Check sheet for the modelled part. Datum: model origin and axes. Units: mm. A direction names the side the tool comes from. Round coordinates to 2 decimals unless told otherwise and drop trailing zeros. Loops run counter-clockwise (first coordinate to the right, second up) from the corner with the lowest first, then second, coordinate; pieces in that order, holes last. Notation, with made-up numbers: M 4.5,35.5 L 61.5,35.5 A16 ccw 61.5,51.5 Z; hole C 45,-5 d9. An arc over 180 degrees is marked long. Write item = value, one per line. Start each with the question number.
(1) Cross-section at A-A on y = 85. Record the boundary of the cut face in (x, z).
(2) Set-up check for faces 1 (the face through (30, 70, -25)), 2 (the face through (300, 32, -199)), 3 (the face through (59, 90, -136)): record each of +Z, -Z, +X, -X, +Y, -Y from which the full face is reachable in a straight line by a thin tool's end or side.
(3) Cross-section at D-D on y = 35.5. Record the boundary of the cut face in (x, z).
(4) Go/stop test with flat-tipped pins: P1, Ø2, axis at y = 103.5, z = -255, coming from the +X side; P2, Ø1, axis at x = 73, y = 66, coming from the +Z side; P3, Ø10, axis at y = 88.5, z = -178, coming from the +X side. Record where each tip stops, or that it passes through.
(5) Scan lines: L1, parallel to Y at x = 205, z = -243; L2, parallel to Z at x = 234.5, y = 84; L3, parallel to Z at x = 75, y = 45.5. Record each from-to range of solid material in increasing order. Write a range as from..to.
(6) Cross-section at B-B on z = -175. Record the boundary of the cut face in (x, y), plus the area to 3 significant figures.
(7) Cross-section at C-C on x = 205. Record the boundary of the cut face in (y, z).
(8) Mould release check, pull along X, two halves, no side actions. Record for faces 4 (the face through (0, 46, -152)), 5 (the face through (154, 92, -225)), 6 (the face through (78.252, 45.63, -189.643)): pulls with the +X half, pulls with the -X half, needs draft (parallel to the pull), parting line crosses it, or undercut.
Autodesk Fusion 360 part; units mm, degrees
sketch "Sketch1" plane through (0, 0, 0) normal (0, 1, 0) x (1, 0, 0)
  line L0 (0, 0) -> (300, 0)
  line L1 (300, 0) -> (300, 300)
  line L2 (300, 300) -> (0, 300)
  line L3 (0, 300) -> (0, 0)
  line L4 (0, 0) -> (200, 0)
  line L5 (300, 300) -> (300, 100)
  line L6 (200, 0) -> (300, 100)
  dimension "d1" = 300
  dimension "d2" = 300
  dimension "d3" = 200
  dimension "d4" = 200
extrude "Extrude1" add sketch "Sketch1" along normal blind 50 contours L0 L1 L2 L3 L4 L5 L6
sketch "Sketch2" plane through (0, 50, 0) normal (0, 1, 0) x (-1, 0, 0)
  line L0 (-300, -300) -> (0, -300)
  line L1 (0, -300) -> (0, 0)
  line L2 (0, 0) -> (-200, 0)
  line L3 (-200, 0) -> (-300, -100)
  line L4 (-300, -100) -> (-300, -300)
  line L5 (0, 0) -> (-30, 0)
  line L6 (-300, -300) -> (-300, -270)
  line L7 (0, -300) -> (0, -270)
  line L8 (0, -300) -> (0, -240)
  line L9 (-300, -270) -> (-255, -225)
  line L10 (0, -300) -> (0, -225)
  line L11 (0, -225) -> (-255, -225)
  line L12 (-30, 0) -> (-30, -50)
  line L13 (-30, -50) -> (-145.4741, -165.4741)
  line L14 (-30, -50) -> (133.305, -50) construction
  line L15 (0, -225) -> (-150, -225)
  line L16 (-150, -225) -> (-150, -170)
  line L17 (-30, -50) -> (-150, -170)
  line L18 (-30, -50) -> (157.6281, -50) construction
  dimension "d7" = 30
  dimension "d8" = 30
  dimension "d9" = 60
  dimension "d11" = 75
  dimension "d12" = 50
  dimension "d13" = 135
  dimension "d14" = 150
  dimension "d15" = 135
extrude "Extrude2" add sketch "Sketch2" along normal blind 40 contours L1 L2 L5 L11 L12 L13 L15 L16 L17
extrude "Extrude3" add sketch "Sketch2" along normal blind 70 contours L0 L1 L4 L6 L7 L8 L9 L10 L11 L15
sketch "Sketch4" plane through (0, 90, 0) normal (0, 1, 0) x (-1, 0, 0)
  line L0 (0, -225) -> (0, 0)
  line L1 (0, 0) -> (-30, 0)
  line L2 (-30, 0) -> (-30, -50)
  line L3 (-30, -50) -> (-150, -170)
  line L4 (-150, -170) -> (-150, -225)
  line L5 (-150, -225) -> (0, -225)
  circle A0 centre (-75, -175) radius 15
  dimension "d20" = 30
  dimension "d21" = 50
  dimension "d22" = 75
extrude "Extrude4" cut sketch "Sketch4" against normal blind 250 contours A0
sketch "Sketch5" plane through (0, 0, -225) normal (0, 0, 1) x (1, 0, 0)
  line L0 (0, 90) -> (150, 90)
  line L1 (150, 90) -> (150, 50)
  line L2 (150, 50) -> (255, 50)
  line L3 (255, 50) -> (255, 120)
  line L4 (255, 120) -> (0, 120)
  line L5 (0, 120) -> (0, 90)
  circle A0 centre (205, 85) radius 15
  dimension "d25" = 30
  dimension "d26" = 35
  dimension "d27" = 55
extrude "Extrude5" cut sketch "Sketch5" against normal blind 410 contours A0
Result:
q1.outline = M 0,-300 L 190,-300 L 190,-225 L 150,-225 L 150,-170 L 30,-50 L 30,0 L 0,0 Z; M 220,-300 L 300,-300 L 300,-270 L 255,-225 L 220,-225 Z; hole C 75,-175 d30
q2.face_1 = +Z, +X, +Y
q2.face_2 = +Z, -Z, +X, +Y, -Y
q2.face_3 = +Z, +X, -X, +Y
q3.outline = M 0,-300 L 300,-300 L 300,-100 L 200,0 L 0,0 Z; hole C 75,-175 d30
q4.P1 = 286
q4.P2 = -92.5
q4.P3 = 150
q5.L1 = 0..70, 100..120
q5.L2 = -300..-225
q5.L3 = -300..-190, -160..0
q6.outline = M 0,0 L 60,0 L 60,90 L 0,90 Z; M 90,0 L 300,0 L 300,50 L 150,50 L 150,90 L 90,90 Z
q6.area = 18,300 mm^2
q7.outline = M 0,-300 L 70,-300 L 70,-225 L 50,-225 L 50,-5 L 0,-5 Z; M 100,-300 L 120,-300 L 120,-225 L 100,-225 Z
q8.face_4 = pulls with the -X half
q8.face_5 = needs draft
q8.face_6 = undercut
